Read the model definition and answer for the solid it produces. Units are mm, in the model's axes. Face numbers are marked on the shaded views. A direction names the side the tool comes from. Coordinates: 2 decimals unless noted, no trailing zeros. Write each loop counter-clockwise with the first axis right and the second up, starting at its lowest first coordinate (ties: lowest second). Pieces come first, ordered by that corner, then holes. Notation, with made-up numbers: (-17, 4.25) - (39, 4.25) arc R31 ccw to (39, 30.25) - close; hole circle Ø7 at (7.5, -25). An arc over 180 degrees is marked (long way). Use a Markdown table: item, result.
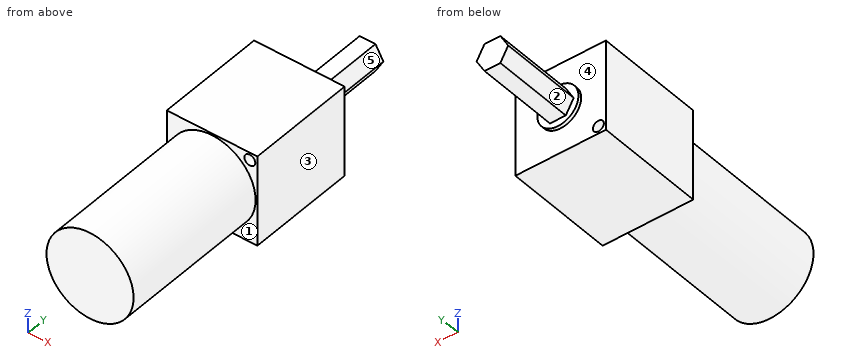
from build123d import *

# Parameters (mm, degrees)
SKETCH1_W           = 42.0116
SKETCH1_H           = 42.0116
SKETCH1_R           = 2.54
BOSS_EXTRUDE1_DEPTH = 50.8
SKETCH2_R           = 9.525
BOSS_EXTRUDE2_DEPTH = 1.5875
BOSS_EXTRUDE3_DEPTH = 38.1
SKETCH4_R           = 20.193
BOSS_EXTRUDE4_DEPTH = 70.993


with BuildPart() as part:
    # Sketch1 → Boss-Extrude1 (new body)
    with BuildSketch(Plane(origin=(0, 0, 0), x_dir=(1, 0, 0), z_dir=(0, 1, 0))):
        Rectangle(SKETCH1_W, SKETCH1_H)
        with Locations((-17.50251918, 17.50251918)):
            Circle(SKETCH1_R, mode=Mode.SUBTRACT)
        with Locations((17.50251918, -17.50251918)):
            Circle(SKETCH1_R, mode=Mode.SUBTRACT)
    extrude(amount=BOSS_EXTRUDE1_DEPTH)

    # Sketch2 → Boss-Extrude2 (add)
    with BuildSketch(Plane(origin=(0, 50.8, 0), x_dir=(1, 0, 0), z_dir=(0, 1, 0))):
        Circle(SKETCH2_R)
    extrude(amount=BOSS_EXTRUDE2_DEPTH)

    # Sketch3 → Boss-Extrude3 (add)
    with BuildSketch(Plane(origin=(0, 52.3875, 0), x_dir=(1, 0, 0), z_dir=(0, 1, 0))):
        Polygon((3.666174209, -6.35), (7.332348419, 0), (3.666174209, 6.35), (-3.666174209, 6.35), (-7.332348419, 0), (-3.666174209, -6.35), align=None)
    extrude(amount=BOSS_EXTRUDE3_DEPTH)

    # Sketch4 → Boss-Extrude4 (add)
    with BuildSketch(Plane.XZ):
        Circle(SKETCH4_R)
    extrude(amount=BOSS_EXTRUDE4_DEPTH)


solid = part.part
(1) A cutting plane is placed at C-C, the plane z = -2.5. Write down the section's boundary in (x, y).
Report:
| item | result |
|---|---|
| outline | (-21.01, 0) - (-20.04, 0) - (-20.04, -70.99) - (20.04, -70.99) - (20.04, 0) - (21.01, 0) - (21.01, 50.8) - (9.19, 50.8) - (9.19, 52.39) - (5.89, 52.39) - (5.89, 90.49) - (-5.89, 90.49) - (-5.89, 52.39) - (-9.19, 52.39) - (-9.19, 50.8) - (-21.01, 50.8) - close |
(2) Each of these flat-tipped pins is pushed along its axis until it touches: P1, Ø6, axis at x = 10.5, y = -9.5, coming from the -Z side; P2, Ø2, axis at x = 0, y = 79, coming from the -Z side; P3, Ø3.5, axis at x = 0, y = 62.5, coming from the +Z side. Where does it stop, or does it pass through?
Report:
| item | result |
|---|---|
| P1 | stops at z = -18.75 |
| P2 | stops at z = -6.35 |
| P3 | stops at z = 6.35 |
(3) Straight lines are drawn through the part: L1, parallel to X at y = 34.5, z = 17.5; L2, parallel to Y at x = 11, z = 10; L3, parallel to X at y = 63, z = -1.5. For each, find the intervals that lie inside material, in ascending order.
Report:
| item | result |
|---|---|
| L1 | x = -21.01 to 14.96, 20.04 to 21.01 |
| L2 | y = -70.99 to 50.8 |
| L3 | x = -6.47 to 6.47 |
(4) A cutting plane is placed at B-B, the plane y = 44. Write down the section's boundary in (x, z).
Report:
| item | result |
|---|---|
| outline | (-21.01, -21.01) - (21.01, -21.01) - (21.01, 21.01) - (-21.01, 21.01) - close; hole circle Ø5.08 at (-17.5, -17.5); hole circle Ø5.08 at (17.5, 17.5) |
(5) For the marked faces 1, 2, 3, 4 and 5, determine the directions among +Z, -Z, +X, -X, +Y, -Y from which every point of the face is accessible in a straight line to the end or side of a thin tool.
Report:
| item | result |
|---|---|
| face 1 | -Y |
| face 2 | -Z, -X, +Y |
| face 3 | +Z, -Z, +X, +Y, -Y |
| face 4 | +Y |
| face 5 | +Z, +X, +Y |
(6) A cutting plane is placed at D-D, the plane y = -26.5. Write down the section's boundary in (x, z).
Report:
| item | result |
|---|---|
| outline | circle Ø40.39 at (0, 0) |
